from build123d import *

# Parameters (mm, degrees)
SKETCH1_R           = 35
BOSS_EXTRUDE1_DEPTH = 10
SKETCH3_R           = 5
CUT_EXTRUDE1_DEPTH  = 5
SKETCH4_R           = 2.5
BOSS_EXTRUDE2_DEPTH = 2


with BuildPart() as part:
    # Sketch1 → Boss-Extrude1 (new body)
    with BuildSketch(Plane(origin=(0, 0, 0), x_dir=(1, 0, 0), z_dir=(0, 1, 0))):
        Circle(SKETCH1_R)
    extrude(amount=BOSS_EXTRUDE1_DEPTH)

    # Sketch2 → Revolve1 (revolve)
    with BuildSketch(Plane(origin=(0, 0, 0), x_dir=(0, 0, -1), z_dir=(1, 0, 0))):
        with BuildLine():
            Line((35, 10), (40, 10))
            Line((40, 10), (40, 7.5))
            Line((40, 7.5), (35.872288151, 6.191567774))
            ThreePointArc((35.872288151, 6.191567774), (35, 5), (35.872288151, 3.808432226))
            Line((35.872288151, 3.808432226), (40, 2.5))
            Line((40, 2.5), (40, 0))
            Line((40, 0), (35, 0))
            Line((35, 0), (34, 0))
            Line((34, 0), (34, 10))
            Line((34, 10), (35, 10))
        make_face()
    revolve(axis=Axis((0, 10, 0), (0, -1, 0)))

    # Sketch3 → Cut-Extrude1 (cut)
    with BuildSketch(Plane.XZ):
        Circle(SKETCH3_R)
    extrude(amount=-CUT_EXTRUDE1_DEPTH, mode=Mode.SUBTRACT)

    # Sketch4 → Boss-Extrude2 (add)
    with BuildSketch(Plane(origin=(0, 10, 0), x_dir=(1, 0, 0), z_dir=(0, 1, 0))):
        with Locations((0, -25)):
            Circle(SKETCH4_R)
    extrude(amount=BOSS_EXTRUDE2_DEPTH)


solid = part.part
CAD build for the part. Positions are in the model's coordinates, mm. A direction names the side the tool comes from. Coordinates: 2 decimals unless noted, no trailing zeros. Write each loop counter-clockwise with the first axis right and the second up, starting at its lowest first coordinate (ties: lowest second). Pieces come first, ordered by that corner, then holes. Notation, with made-up numbers: M 15,-21 L 71,-21 A28 cw 71,8 Z; hole C -30,-23 d9. An arc over 180 degrees is marked long. Answer as a JSON object with one key per item and string values. Group by question number.
1) Tool access for faces 1 (the face through (10.853, 3.727, -34.462)), 2 (the face through (-1.08, 2.46, -4.88)), 3 (the face through (-39.05, 1.23, 8.67)): list every direction of +Z, -Z, +X, -X, +Y, -Y with a clear straight run to the whole face (end or side of a thin tool).
2) Wall check: line 1 (Y direction, x = 34.5, z = 10); line 2 (Y direction, x = -20.5, z = 28.5); line 3 (X direction, y = 0.5, z = -0.5). Give the ranges that are in metal, low to high. Write a range as from..to.
3) Saw through at A-A (x = 0). Write the cut outline in (y, z).
4) Saw through at C-C (y = 11). Write the cut outline in (x, z), plus the area to 3 significant figures.
5) Saw through at B-B (z = 0). Write the cut outline in (x, y).
6) Mould opens along Y. For faces 4 (the face through (1, 0, -8)), 5 (the face through (-35.215, 6.255, 7.82)), 6 (the face through (0, 12, 25)), 7 (the face through (-0.33, 10.99, 22.52)) say: +Y half, -Y half, draft (parallel to the pull), parting line (faces both ways), or undercut.
7) Pin check, flat tips, straight feed: pin 1 Ø2 at (x, y) = (15.5, 10) entering from -Z; pin 2 Ø5 at (x, z) = (26.5, 7) entering from +Y; pin 3 Ø6 at (x, y) = (-5, 9.5) entering from -Z. Stop position of each tip, or through.
Values follow:
{
 "1": {"face 1": "none", "face 2": "-Y", "face 3": "+Y, -Y"},
 "2": {"line 1": "y = 0..3.79, 6.21..10", "line 2": "y = 0..4.49, 5.51..10", "line 3": "x = -40..-4.97, 4.97..40"},
 "3": {"outline": "M 0,-40 L 2.5,-40 L 3.81,-35.87 A1.25 cw 6.19,-35.87 L 7.5,-40 L 10,-40 L 10,22.5 L 12,22.5 L 12,27.5 L 10,27.5 L 10,40 L 7.5,40 L 6.19,35.87 A1.25 cw 3.81,35.87 L 2.5,40 L 0,40 L 0,5 L 5,5 L 5,-5 L 0,-5 Z"},
 "4": {"outline": "C 0,25 d5", "area": "19.6 mm2"},
 "5": {"outline": "M -40,0 L -5,0 L -5,5 L 5,5 L 5,0 L 40,0 L 40,2.5 L 35.87,3.81 A1.25 cw 35.87,6.19 L 40,7.5 L 40,10 L -40,10 L -40,7.5 L -35.87,6.19 A1.25 cw -35.87,3.81 L -40,2.5 Z"},
 "6": {"face 4": "-Y half", "face 5": "undercut", "face 6": "+Y half", "face 7": "draft"},
 "7": {"pin 1": "stops at z = -37.28", "pin 2": "stops at y = 10", "pin 3": "stops at z = -39.95"}
}
